Geometry: final body of the model. Coordinates: model frame, mm. A direction names the side the tool comes from. Coordinates: 2 decimals unless noted, no trailing zeros. Write each loop counter-clockwise with the first axis right and the second up, starting at its lowest first coordinate (ties: lowest second). Pieces come first, ordered by that corner, then holes.
from build123d import *
from OCP.BRepFilletAPI import BRepFilletAPI_MakeChamfer

# Parameters (mm, degrees)
SKIZZE1_W                            = 4.6
SKIZZE1_H                            = 10.4
SKIZZE1_W_2                          = 11.1
SKIZZE1_H_2                          = 50
SKIZZE1_H_3                          = 6.7
SKIZZE1_H_4                          = 8.8
AUFSATZ_LINEAR_AUSTRAGEN1_DEPTH      = 3
SCHNITT_LINEAR_AUSTRAGEN1_DEPTH      = 37.5
SCHNITT_LINEAR_AUSTRAGEN1_DEPTH_BACK = 67.5
SKIZZE2_R                            = 1
SKIZZE3_W                            = 5.1
SKIZZE3_H                            = 22
SCHNITT_LINEAR_AUSTRAGEN2_DEPTH      = 7.5
VERRUNDUNG4_R                        = 1
SKIZZE4_W                            = 2
SKIZZE4_H                            = 9.5
SCHNITT_LINEAR_AUSTRAGEN3_DEPTH      = 1
VERRUNDUNG5_R                        = 1
SKIZZE7_W                            = 8.5
SKIZZE7_H                            = 0.94
SKIZZE7_W_2                          = 1.53828676
SKIZZE7_H_2                          = 8.4
SKIZZE7_H_3                          = 4.7
SKIZZE7_H_4                          = 6.8
AUFSATZ_LINEAR_AUSTRAGEN4_DEPTH      = 1
FASE1_SIZE                           = 1.6
FASE1_SIZE2                          = 0.582352375


with BuildPart() as part:
    # Skizze1 → Aufsatz-Linear austragen1 (new body)
    with BuildSketch(Plane.XY):
        with Locations((-18, 14.120550309)):
            Rectangle(SKIZZE1_W, SKIZZE1_H)
        with Locations((-10.15, 24.220550309)):
            Rectangle(SKIZZE1_W_2, SKIZZE1_H_2)
        with Locations((-18, 34.320550309)):
            Rectangle(SKIZZE1_W, SKIZZE1_H)
        with Locations((-2.3, 43.370550309)):
            Rectangle(SKIZZE1_W, SKIZZE1_H_3)
        with Locations((-2.3, 5.070550309)):
            Rectangle(SKIZZE1_W, SKIZZE1_H_3)
        with Locations((-2.3, 24.220550309)):
            Rectangle(SKIZZE1_W, SKIZZE1_H_4)
    extrude(amount=AUFSATZ_LINEAR_AUSTRAGEN1_DEPTH)

    # Skizze2 → Schnitt-Linear austragen1 (cut, two sides: drawn at the far end of the back side and taken through both)
    with BuildSketch(Plane(origin=(0, 39.520550309, 0), x_dir=(1, 0, 0), z_dir=(0, 1, 0)).offset(-SCHNITT_LINEAR_AUSTRAGEN1_DEPTH_BACK)):
        with Locations(Location((-18.3, -1.5, 0), (0, 0, 270))):
            Circle(SKIZZE2_R)
        with Locations(Location((-2, -1.5, 0), (0, 0, 90))):
            Circle(SKIZZE2_R)
    extrude(amount=SCHNITT_LINEAR_AUSTRAGEN1_DEPTH + SCHNITT_LINEAR_AUSTRAGEN1_DEPTH_BACK, mode=Mode.SUBTRACT)

    # Skizze3 → Schnitt-Linear austragen2 (cut)
    with BuildSketch(Plane.XY.offset(3)):
        with Locations((-10.15, 24.220550309)):
            Rectangle(SKIZZE3_W, SKIZZE3_H)
    extrude(amount=-SCHNITT_LINEAR_AUSTRAGEN2_DEPTH, mode=Mode.SUBTRACT)

    # Verrundung4
    verrundung4_edges = [part.edges().sort_by_distance(p)[0] for p in [
        (-20.3, 14.120550309, 3),
        (-20.3, 34.320550309, 3),
        (-20.3, 34.320550309, 0),
        (0, 43.370550309, 0),
        (0, 24.220550309, 0),
        (0, 5.070550309, 0),
        (-20.3, 14.120550309, 0),
        (0, 5.070550309, 3),
        (0, 24.220550309, 3),
        (0, 43.370550309, 3),
    ]]
    fillet(verrundung4_edges, radius=VERRUNDUNG4_R)

    # Skizze4 → Schnitt-Linear austragen3 (cut)
    with BuildSketch(Plane.XY.offset(3)):
        with Locations((-12.5, 42.470550309)):
            Rectangle(SKIZZE4_W, SKIZZE4_H)
        with Locations((-12.5, 5.970550309)):
            Rectangle(SKIZZE4_W, SKIZZE4_H)
        with Locations((-7.8, 42.470550309)):
            Rectangle(SKIZZE4_W, SKIZZE4_H)
        with Locations((-7.8, 5.970550309)):
            Rectangle(SKIZZE4_W, SKIZZE4_H)
    extrude(amount=-SCHNITT_LINEAR_AUSTRAGEN3_DEPTH, mode=Mode.SUBTRACT)

    # Verrundung5
    verrundung5_edges = [part.edges().sort_by_distance(p)[0] for p in [
        (-6.8, 5.970550309, 2),
        (-13.5, 5.970550309, 2),
        (-13.5, 42.470550309, 2),
        (-6.8, 42.470550309, 2),
    ]]
    fillet(verrundung5_edges, radius=VERRUNDUNG5_R - 0.0001)  # a hair under: the kernel refuses the full size

    # Skizze7 → Aufsatz-Linear austragen4 (add)
    with BuildSketch(Plane.XY.offset(3)):
        with Locations((-10.7, 48.220550309)):
            Rectangle(SKIZZE7_W, SKIZZE7_H)
        with Locations((-10.15, 0.220550309)):
            Rectangle(SKIZZE7_W, SKIZZE7_H)
        with Locations((-15.385238006, 14.120550309)):
            Rectangle(SKIZZE7_W_2, SKIZZE7_H_2)
        with Locations((-2.685428708, 5.070550309)):
            Rectangle(SKIZZE7_W_2, SKIZZE7_H_3)
        with Locations((-2.685428708, 24.220550309)):
            Rectangle(SKIZZE7_W_2, SKIZZE7_H_4)
        with Locations((-15.385238006, 34.320550309)):
            Rectangle(SKIZZE7_W_2, SKIZZE7_H_2)
        with Locations((-2.685428708, 43.370550309)):
            Rectangle(SKIZZE7_W_2, SKIZZE7_H_3)
    extrude(amount=AUFSATZ_LINEAR_AUSTRAGEN4_DEPTH)

    # Fase1: one chamfer whose edges measure the first distance from different faces: ONE call of the kernel's chamfer builder (chamfer() names one face for all edges)
    fase1_edges_1 = [part.edges().sort_by_distance(p)[0] for p in [
        (-10.15, 35.220550309, 0),
    ]]
    fase1_side_1 = [part.faces().sort_by_distance(p)[0] for p in [
        (-10.15, 35.220550309, 1.5),
    ]]
    fase1_edges_2 = [part.edges().sort_by_distance(p)[0] for p in [
        (-12.7, 24.220550309, 0),
    ]]
    fase1_side_2 = [part.faces().sort_by_distance(p)[0] for p in [
        (-12.7, 24.220550309, 1.5),
    ]]
    fase1_edges_3 = [part.edges().sort_by_distance(p)[0] for p in [
        (-10.15, 13.220550309, 0),
    ]]
    fase1_side_3 = [part.faces().sort_by_distance(p)[0] for p in [
        (-10.15, 13.220550309, 1.5),
    ]]
    fase1_edges_4 = [part.edges().sort_by_distance(p)[0] for p in [
        (-7.6, 24.220550309, 0),
    ]]
    fase1_side_4 = [part.faces().sort_by_distance(p)[0] for p in [
        (-7.6, 24.220550309, 1.5),
    ]]
    fase1 = BRepFilletAPI_MakeChamfer(part.part.solid().wrapped)
    for e in fase1_edges_1:
        fase1.Add(FASE1_SIZE, FASE1_SIZE2, e.wrapped, fase1_side_1[0].wrapped)  # the first distance lies on this face
    for e in fase1_edges_2:
        fase1.Add(FASE1_SIZE, FASE1_SIZE2, e.wrapped, fase1_side_2[0].wrapped)  # the first distance lies on this face
    for e in fase1_edges_3:
        fase1.Add(FASE1_SIZE, FASE1_SIZE2, e.wrapped, fase1_side_3[0].wrapped)  # the first distance lies on this face
    for e in fase1_edges_4:
        fase1.Add(FASE1_SIZE, FASE1_SIZE2, e.wrapped, fase1_side_4[0].wrapped)  # the first distance lies on this face
    add(Compound.cast(fase1.Shape()), mode=Mode.REPLACE)


solid = part.part
Item 1: Pin query (flat end, axial travel): pin 1 (0.7 mm diameter, centred on y = 27, z = 2, fed in from -X); pin 2 (0.8 mm diameter, centred on y = 5.5, z = 3.5, fed in from +X); pin 3 (1 mm diameter, centred on x = -4.5, y = 36.5, fed in from +Z); pin 4 (1.2 mm diameter, centred on x = -2, z = 1.5, fed in from -Y). Return the tip coordinate at first contact, or that it passes through.
Derived:
pin 1: stops at x = -15.7
pin 2: stops at x = -1.92
pin 3: stops at z = 3
pin 4: passes through
Item 2: Section C-C, the plane x = -18.3. Output: boundary loops of the cut face in (y, z), plus the area to 3 significant figures.
Derived:
outline: (8.92, 0) - (19.32, 0) - (19.32, 0.5) - (8.92, 0.5) - close; (8.92, 2.5) - (19.32, 2.5) - (19.32, 3) - (8.92, 3) - close; (29.12, 0) - (39.52, 0) - (39.52, 0.5) - (29.12, 0.5) - close; (29.12, 2.5) - (39.52, 2.5) - (39.52, 3) - (29.12, 3) - close
area: 20.8 mm2
Item 3: Pull-direction query (X, two-part tool) for faces 4 (the flat face through (-16.154, 34.3, 3.5)), 5 (the cylindrical face through (-1.024, 43.324, 1.717)), 6 (the flat face through (-14.616, 34.3, 3.5)); classes: released by +X, released by -X, zero draft, split by the parting line, or undercut.
Derived:
face 4: released by -X
face 5: undercut
face 6: released by +X
Item 4: Section D-D, the plane y = 36.5. Output: boundary loops of the cut face in (x, z), plus the area to 3 significant figures.
Derived:
outline: (-20.3, 1) arc R1 ccw to (-19.3, 0) - (-4.6, 0) - (-4.6, 3) - (-14.62, 3) - (-14.62, 4) - (-16.15, 4) - (-16.15, 3) - (-19.3, 3) arc R1 ccw to (-20.3, 2) - close; hole circle Ø2 at (-18.3, 1.5)
area: 45.1 mm2
Item 5: Section A-A, the plane y = 22. Output: boundary loops of the cut face in (x, z), plus the area to 3 significant figures.
Derived:
outline: (-15.7, 0) - (-13.28, 0) - (-12.7, 1.6) - (-12.7, 3) - (-15.7, 3) - close; (-7.6, 1.6) - (-7.02, 0) - (-1, 0) arc R1 ccw to (0, 1) - (0, 2) arc R1 ccw to (-1, 3) - (-1.92, 3) - (-1.92, 4) - (-3.45, 4) - (-3.45, 3) - (-7.6, 3) - close; hole circle Ø2 at (-2, 1.5)
area: 28.8 mm2
Item 6: Material intervals for probe 1 along X at (y, z) = (44, 1.55); probe 2 along Y at (x, z) = (-11.75, 3.25); probe 3 along Y at (x, z) = (-2.75, 2.6), sorted ascending.
Derived:
probe 1: x = -15.7 to -3, -1 to 0
probe 2: y = -0.25 to 0.69, 47.75 to 48.69
probe 3: y = 1.72 to 8.42, 19.82 to 28.62, 40.02 to 46.72
Item 7: Set-up query: faces 1 (the flat face through (-6.45, 48.2, 3.5)), 2 (the flat face through (-12.995, 24.058, 0.789)), 3 (the flat face through (-3.455, 24.2, 3.5)). Return all of +Z, -Z, +X, -X, +Y, -Y with unobstructed straight access to the full face (end or side cutting, diameter ignored); none if empty.
Derived:
face 1: +Z, +X, +Y
face 2: -Z
face 3: +Z, -X, +Y, -Y
